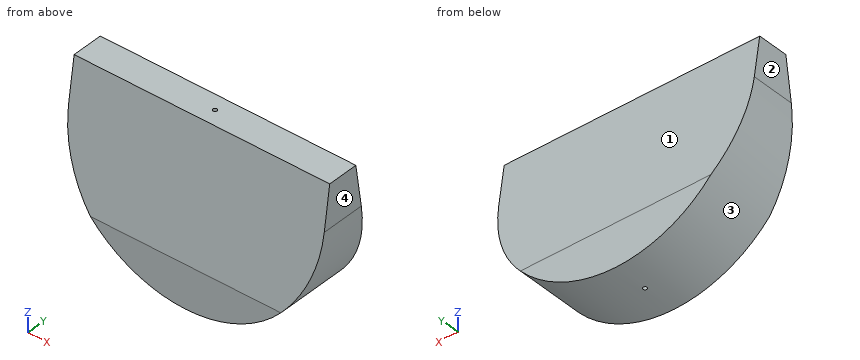
Autodesk Inventor part; units mm, degrees
ref_plane "YZ Plane" through (0, 0, 0) normal (1, 0, 0) x (0, 1, 0)
ref_plane "XZ Plane" through (0, 0, 0) normal (0, 1, 0) x (-1, 0, 0)
ref_plane "XY Plane" through (0, 0, 0) normal (0, 0, 1) x (1, 0, 0)
sketch "Эскиз1" plane through (0, 0, 0) normal (0, 1, 0) x (-1, 0, 0)
  line L0 (165, 0.2529) -> (-165, 0.2529)
  line L1 (-165, 0.2529) -> (-165, -54.7471)
  line L2 (165, 0.2529) -> (165, -54.7471)
  arc A0 (-165, -54.7471) -> (165, -54.7471) centre (0, -54.7471) ccw
  point P0 (0, 0)
  dimension "d1" = 330
  dimension "d5" = 55
  dimension "d8" = 55
extrude "Выдавливание1" add sketch "Эскиз1" along normal mid plane 90
sketch "Эскиз2" plane through (0, 0, 0) normal (1, 0, 0) x (0, 1, 0)
  line L0 (-45, -54.7471) -> (45, -54.7471)
  line L1 (45, 0.2529) -> (45, -54.7471)
  line L2 (0, -101.1017) -> (0, -121.0064)
  line L3 (-20, -219.7471) -> (-45, -54.7471)
  line L4 (20, 0.2529) -> (45, -164.7471)
  line L5 (45, 0.2529) -> (20, 0.2529)
  line L6 (45, 0.2529) -> (45, -164.7471)
  line L7 (-45, 0.2529) -> (-45, -54.7471)
  line L8 (-20, 0.2529) -> (-45, -164.7471)
  line L9 (-45, 0.2529) -> (-20, 0.2529)
  line L10 (-45, 0.2529) -> (-45, -164.7471)
  point P0 (0, 0)
extrude "Выдавливание2" cut sketch "Эскиз2" along normal mid plane 330
sketch "Эскиз3" plane through (-165, -20, 0.2529) normal (0, 0, 1) x (1, 0, 0)
  circle A0 centre (165, 20) radius 2.65
  dimension "d14" = 5.3
extrude "Выдавливание3" cut sketch "Эскиз3" against normal up to surface
properties part number "Сыр"
Geometry check sheet. Reference: the model listing, model coordinates, mm. Face numbers are marked on the shaded views. Coordinates: 2 decimals unless noted, no trailing zeros. Loops run counter-clockwise (first coordinate to the right, second up) from the corner with the lowest first, then second, coordinate; pieces in that order, holes last. Notation, with made-up numbers: (56.25, 7.5) -> (106.25, 7.5) arc R23 cw to (106.25, 16.5) -> close; hole circle Ø7 at (7, 69.5). An arc over 180 degrees is marked (long way). Put each result on its own line as item: value.
1) Cross-section at D-D on x = -48. Record the boundary of the cut face in (y, z), plus the area to 3 significant figures.
Result set:
outline: (-45, -212.61) -> (45, -212.61) -> (45, -164.75) -> (20, 0.25) -> (-20, 0.25) -> (-45, -164.75) -> close
area: 15,000 mm^2
2) Cross-section at B-B on z = -51. Record the boundary of the cut face in (x, y).
Result set:
outline: (-165, -27.77) -> (165, -27.77) -> (165, 27.77) -> (-165, 27.77) -> close; hole circle Ø5.3 at (0, 0)
3) Release check for a two-part mould opening along X. For the marked faces 1, 2, 3 and 4 record: released by +X, released by -X, zero draft, split by the parting line, or undercut.
Result set:
face 1: zero draft
face 2: released by -X
face 3: split by the parting line
face 4: released by +X
4) Gauge pin test, flat ends, axial feed: pin 1 Ø8 at (x, y) = (104, 31.5) entering from -Z; pin 2 Ø6 at (y, z) = (15, -168.5) entering from -X; pin 3 Ø10 at (x, z) = (66.5, -50.5) entering from +Y. Record the tip position at first contact, or that the pin passes through.
Result set:
pin 1: stops at z = -185.99
pin 2: stops at x = -122.31
pin 3: stops at y = 28.45
5) Cross-section at A-A on x = -87. Record the boundary of the cut face in (y, z), plus the area to 3 significant figures.
Result set:
outline: (-45, -194.95) -> (45, -194.95) -> (45, -164.75) -> (20, 0.25) -> (-20, 0.25) -> (-45, -164.75) -> close
area: 13,400 mm^2
6) Thickness scan on line 1 (Y direction, x = 0, z = -120.5); line 2 (Y direction, x = 1.5, z = -101.5); line 3 (Z direction, x = 4, y = 6). Record the ranges inside material, lowest first.
Result set:
line 1: y = -38.3 to -2.65, 2.65 to 38.3
line 2: y = -35.42 to -2.18, 2.18 to 35.42
line 3: z = -219.7 to 0.25
7) Cross-section at C-C on y = 13.5. Record the boundary of the cut face in (x, z), plus the area to 3 significant figures.
Result set:
outline: (-165, -54.75) arc R165 ccw to (165, -54.75) -> (165, 0.25) -> (-165, 0.25) -> close
area: 60,900 mm^2
